Part model, mm, in its own coordinate system. A direction names the side the tool comes from. Coordinates: 2 decimals unless noted, no trailing zeros. Loops run counter-clockwise (first coordinate to the right, second up) from the corner with the lowest first, then second, coordinate; pieces in that order, holes last. Notation, with made-up numbers: M 8.25,61 L 45.25,61 A16 ccw 45.25,76 Z; hole C 72.25,41.25 d7. An arc over 180 degrees is marked long. Use CSV: the item, a comma, the result in double quotes. Start each with the question number.
from build123d import *

# Parameters (mm, degrees)
F0_W      = 35
F0_H      = 26
F0_R      = 1.2
F1_DEPTH  = 2.5
F2_R      = 3
F3_DEPTH  = 3
F3_FACE_R = 1.2
F4_DEPTH  = 25
F5_DEPTH  = 25
F6_W      = 20
F6_H      = 2.5
F7_DEPTH  = 9


with BuildPart() as f1:
    # F0 (on Top) → F1 (new body)
    with BuildSketch(Plane.XY):
        with Locations((2.61107, 5.940669)):
            Rectangle(F0_W, F0_H)
        with Locations((-3.88893, 5.940669)):
            Circle(F0_R, mode=Mode.SUBTRACT)
        with Locations((15.11107, 5.940669)):
            Circle(F0_R, mode=Mode.SUBTRACT)
    extrude(amount=F1_DEPTH)

    # F2 (on face) → F3 (join)
    with BuildSketch(Plane(origin=(0, 0, 0), x_dir=(1, 0, 0), z_dir=(0, 0, -1))):
        with Locations((-3.88893, -5.940669)):
            Circle(F2_R)
        with Locations((15.11107, -5.940669)):
            Circle(F2_R)
    extrude(amount=F3_DEPTH)

    # F3_face (on face) → F4 (cut)
    with BuildSketch(Plane(origin=(-3.88893, 5.940669, 0), x_dir=(1, 0, 0), z_dir=(0, 0, 1))):
        Circle(F3_FACE_R)
    extrude(amount=-F4_DEPTH, mode=Mode.SUBTRACT)

    # F3_face (on face) → F5 (cut)
    with BuildSketch(Plane(origin=(-3.88893, 5.940669, 0), x_dir=(1, 0, 0), z_dir=(0, 0, 1))):
        with Locations((19, 0)):
            Circle(F3_FACE_R)
    extrude(amount=-F5_DEPTH, mode=Mode.SUBTRACT)

    # F6 (on face) → F7 (join)
    with BuildSketch(Plane(origin=(-14.88893, 0, 0), x_dir=(0, -1, 0), z_dir=(-1, 0, 0))):
        with Locations((-8.940669, 1.25)):
            Rectangle(F6_W, F6_H)
    extrude(amount=F7_DEPTH)


solid = f1.part
1. Slice it at B-B, the plane x = -6. List the corners of the cut face in (y, z), and give its area (3 significant figures).
2. Slice it at A-A, the plane z = 0.9. List the corners of the cut face in (x, y), and give its area (3 significant figures).
3. Tool access for faces 5 (the face through (-19, -1.059, 1)), 6 (the face through (-2, 18.941, 1)): list every direction of +Z, -Z, +X, -X, +Y, -Y with a clear straight run to the whole face (end or side of a thin tool).
4. Pin check, flat tips, straight feed: pin 1 (1.2 mm diameter, centred on x = -20, z = 1, fed in from -Y); pin 2 (1.9 mm diameter, centred on x = 15.11, y = 5.94, fed in from +Z); pin 3 (1 mm diameter, centred on x = 11.5, y = -3.5, fed in from -Z); pin 4 (2 mm diameter, centred on y = -4.5, z = 1, fed in from -X). Stop position of each tip, or through.
5. Wall check: probe 1 along X at (y, z) = (5.5, -0.85); probe 2 along Z at (x, y) = (3, -5.5); probe 3 along X at (y, z) = (6.75, 1.2). Give the ranges that are in metal, low to high.
6. Slice it at D-D, the plane z = -0.9. List the corners of the cut face in (x, y), and give its area (3 significant figures).
7. Two-plate mould, pull along X, no slides. Class faces 1 (the face through (-14.889, -4, 1)), 2 (the face through (-2.28, 3.41, -1.48)), 3 (the face through (-2, 6, 2.5)), 4 (the face through (12.9, 3.913, -1.479)): pulls with the +X half, pulls with the -X half, needs draft (parallel to the pull), parting line crosses it, or undercut.
8. Slice it at C-C, the plane y = 15.75. List the corners of the cut face in (x, z).
Found:
1,outline,"M -7.06,0 L 3.81,0 L 3.81,-3 L 8.07,-3 L 8.07,0 L 18.94,0 L 18.94,2.5 L -7.06,2.5 Z"
1,area,"77.8 mm^2"
2,outline,"M -23.89,-1.06 L -14.89,-1.06 L -14.89,-7.06 L 20.11,-7.06 L 20.11,18.94 L -23.89,18.94 Z; hole C -3.89,5.94 d2.4; hole C 15.11,5.94 d2.4"
2,area,"1,080 mm^2"
3,face 5,"+Z, -Z, -X, -Y"
3,face 6,"+Z, -Z, +X, -X, +Y"
4,pin 1,"y = -1.06"
4,pin 2,"through"
4,pin 3,"z = 0"
4,pin 4,"x = -14.89"
5,probe 1,"-6.86 to -5.01, -2.77 to -0.92, 12.14 to 13.99, 16.23 to 18.08"
5,probe 2,"0 to 2.5"
5,probe 3,"-23.89 to -4.77, -3 to 14.23, 16 to 20.11"
6,outline,"C -3.89,5.94 d6; C 15.11,5.94 d6; hole C -3.89,5.94 d2.4; hole C 15.11,5.94 d2.4"
6,area,"47.5 mm^2"
7,face 1,"pulls with the -X half"
7,face 2,"undercut"
7,face 3,"needs draft"
7,face 4,"undercut"
8,outline,"M -23.89,0 L 20.11,0 L 20.11,2.5 L -23.89,2.5 Z"
